Autodesk Inventor part; units mm, degrees
ref_plane "YZ Plane" through (0, 0, 0) normal (1, 0, 0) x (0, 1, 0)
ref_plane "XZ Plane" through (0, 0, 0) normal (0, 1, 0) x (-1, 0, 0)
ref_plane "XY Plane" through (0, 0, 0) normal (0, 0, 1) x (1, 0, 0)
sketch "Sketch1" plane through (0, 0, 0) normal (0, 0, 1) x (1, 0, 0)
  line L0 (-9.525, -66.675) -> (9.525, -66.675)
  line L1 (9.525, -66.675) -> (9.525, 66.675)
  line L2 (9.525, 66.675) -> (-9.525, 66.675)
  line L3 (-9.525, 66.675) -> (-9.525, -66.675)
  line L4 (-9.525, -66.675) -> (9.525, 66.675) construction
  line L5 (9.525, -66.675) -> (-9.525, 66.675) construction
  point P0 (0, 0)
  dimension "d0" = 19.05
  dimension "d1" = 133.35
extrude "Extrusion1" add sketch "Sketch1" along normal blind 6.35
sketch "Sketch4" plane through (0, 0, 6.35) normal (0, 0, 1) x (1, 0, 0)
  line L0 (1.6891, -57.15) -> (-1.6891, -57.15)
  line L1 (-1.6891, -57.15) -> (-1.6891, 57.15)
  line L2 (-1.6891, 57.15) -> (1.6891, 57.15)
  line L3 (1.6891, 57.15) -> (1.6891, -57.15)
  line L4 (1.6891, -57.15) -> (-1.6891, 57.15) construction
  line L5 (-1.6891, -57.15) -> (1.6891, 57.15) construction
  point P0 (0, 0)
  dimension "d16" = 3.3782
  dimension "d17" = 114.3
extrude "Extrusion3" cut sketch "Sketch4" against normal through all
fillet "Fillet2" radius 1.6891 4 edges at (-1.6891, 57.15, 3.175) (1.6891, 57.15, 3.175) (-1.6891, -57.15, 3.175) (1.6891, -57.15, 3.175)
sketch "Sketch5" plane through (0, 0, 6.35) normal (0, 0, 1) x (1, 0, 0)
  line L0 (-3.175, -58.6359) -> (3.175, -58.6359)
  line L1 (3.175, -58.6359) -> (3.175, 58.6359)
  line L2 (3.175, 58.6359) -> (-3.175, 58.6359)
  line L3 (-3.175, 58.6359) -> (-3.175, -58.6359)
  line L4 (-3.175, -58.6359) -> (3.175, 58.6359) construction
  line L5 (3.175, -58.6359) -> (-3.175, 58.6359) construction
  line L6 (1.6891, 55.4609) -> (1.6891, -55.4609)
  arc A0 (-1.6891, -55.4609) -> (1.6891, -55.4609) centre (0, -55.4609) ccw
  line L7 (-1.6891, -55.4609) -> (-1.6891, 55.4609)
  arc A1 (1.6891, 55.4609) -> (-1.6891, 55.4609) centre (0, 55.4609) ccw
  line L8 (-9.525, -66.675) -> (9.525, -66.675)
  line L9 (9.525, -66.675) -> (9.525, 66.675)
  line L10 (9.525, 66.675) -> (-9.525, 66.675)
  line L11 (-9.525, 66.675) -> (-9.525, -66.675)
  line L12 (-3.175, -58.6359) -> (3.175, -52.2859)
  point P0 (0, 0)
  dimension "d21" = 6.35
  dimension "d31" = 45
extrude "Extrusion4" cut sketch "Sketch5" against normal blind 3.175 contours L12 A0 L6 L1 L0 | L3 L2 L1 L12 L6 A1 L7 A0
fillet "Fillet3" radius 3.175 4 edges at (-3.175, -58.6359, 4.7625) (3.175, -58.6359, 4.7625) (3.175, 58.6359, 4.7625) (-3.175, 58.6359, 4.7625)
equation "\"d0\" = sensorHolderDepth"
equation "\"d1\" = width + internalAcrylicThickness"
equation "\"d2\" = acrylicThickness"
equation "\"d17\" = width - 2 * acrylicThickness"
equation "\"d18\" = acrylicThickness"
equation "\"acrylicThickness\" = 6.35"
equation "\"height\" = 127"
equation "\"width\" = 127"
equation "\"depth\" = 127"
equation "\"mirrorAngle\" = 5deg"
equation "\"detectorWidth\" = 52"
equation "\"detectorHeight\" = 52"
equation "\"mirrorThickness\" = 3.175"
equation "\"fresnelThickness\" = 0.1"
equation "\"focalLength\" = 76.2"
equation "\"ior\" = 1.49"
equation "\"centerThickness\" = 1.524"
equation "\"fresnelAngle\" = 90deg"
equation "\"fresnelEffectiveDiameter\" = 152.4"
equation "\"mirrorSuppourtWidth\" = 38.1"
equation "\"backGrooveBit\" = 4.8006"
equation "\"detectorOpeningWidth\" = 76.2"
equation "\"detectorOpeningHeight\" = 76.2"
equation "\"sensorHolderSensorHeight\" = 53.975"
equation "\"sensorHolderSensorWidth\" = 53.975"
equation "\"oRingWidth\" = 1.5875"
equation "\"sensorHolderORingID\" = 203.2"
equation "\"sensorHolderFlushORingID\" = 304.8"
equation "\"frontBackORingID\" = 419.1"
equation "\"mirrorGroove\" = 19.05"
equation "\"backMirrorGroove\" = 6.35"
equation "\"fresnelMirrorChamfer\" = 6.35"
equation "\"mirrorGrooveMill\" = 3.175"
equation "\"sensorHolderDepth\" = 19.05"
equation "\"internalAcrylicThicnkess\" = 6.35"
equation "\"frameAcrylicThickness\" = 9.525"
equation "\"internalAcrylicThickness\" = 6.35"
equation "\"aerogelClearence\" = 3.175"
equation "\"backplanePostionOffsett\" = 12.7"
equation "\"backplanePCBWidth\" = 76.2"
equation "\"backplanePCBHeight\" = 76.2"
equation "\"backplaneHoleOffsett\" = 6.35"
equation "\"moduleSlotClearence\" = 0.79375"
equation "\"plasticThickness\" = 6.35"
equation "\"aerogelHolderDepth\" = 37.30625"
properties part number "horizontalSupourt" material "ABS Plastic"
Work out the finished part from the listing and answer in its coordinate system (mm). A direction names the side the tool comes from. Coordinates: 2 decimals unless noted, no trailing zeros. Write each loop counter-clockwise with the first axis right and the second up, starting at its lowest first coordinate (ties: lowest second). Pieces come first, ordered by that corner, then holes. Notation, with made-up numbers: M -19,31.25 L -2,31.25 A20 cw -2,65.25 Z; hole C 71,80 d2. An arc over 180 degrees is marked long. Write item = value, one per line.
1. The part is cut by section A-A (y = 35). Determine the outline of the cut face in (x, z) (3 decimals), then the cut area to 3 significant figures.
Solution:
outline = M -9.525,0 L -1.689,0 L -1.689,3.175 L -3.175,3.175 L -3.175,6.35 L -9.525,6.35 Z; M 1.689,0 L 9.525,0 L 9.525,6.35 L 3.175,6.35 L 3.175,3.175 L 1.689,3.175 Z
area = 90.1 mm2
2. A flat-ended cylindrical pin translates along its axis: pin 1 (5 mm diameter, centred on x = -0.5, y = 18.5, fed in from +Z) (3 decimals). Find the tip coordinate at first contact, or state that the pin passes through.
Solution:
pin_1 = 3.175
3. Straight lines are drawn through the part: line 1 (X direction, y = -44, z = 1.5) (3 decimals); line 2 (X direction, y = -49.5, z = 6) (3 decimals); line 3 (Z direction, x = 3, y = -10) (3 decimals). For each, find the intervals that lie inside material, in ascending order. Write a range as from..to.
Solution:
line_1 = -9.525..-1.689, 1.689..9.525
line_2 = -9.525..-3.175, 3.175..9.525
line_3 = 0..3.175
4. Determine the mould class of faces 4 (the face through (-1.689, -1, 2)), 5 (the face through (-2.22, -57.73, 4.74)), 6 (the face through (4, 1, 6.35)), 7 (the face through (0, -66.675, 3)) for opening direction Y: released by +Y, released by -Y, zero draft, split by the parting line, or undercut.
Solution:
face_4 = undercut
face_5 = undercut
face_6 = zero draft
face_7 = released by -Y
5. For faces 1 (the face through (-3.175, 1, 5)), 2 (the face through (1.689, 1, 2)), 3 (the face through (0, 66.675, 3)), determine the directions among +Z, -Z, +X, -X, +Y, -Y from which every point of the face is accessible in a straight line to the end or side of a thin tool.
Solution:
face_1 = +Z
face_2 = +Z, -Z
face_3 = +Z, -Z, +X, -X, +Y
